Model file for the job. Use its own axes, mm. Round coordinates to 2 decimals unless told otherwise and drop trailing zeros. Loops run counter-clockwise (first coordinate to the right, second up) from the corner with the lowest first, then second, coordinate; pieces in that order, holes last. Notation, with made-up numbers: (59.25, 9.5) - (87.25, 9.5) arc R16 ccw to (87.25, 19.5) - close; hole circle Ø6 at (12.5, -1.75). An arc over 180 degrees is marked (long way). Answer as a JSON object with one key per item and string values.
from build123d import *

# Parameters (mm, degrees)
BOSS_EXTRUDE1_DEPTH = 3.175
CUT_EXTRUDE1_REACH  = 5.175
SKETCH2_R           = 7.14375
SKETCH3_R           = 6.35
CUT_EXTRUDE2_DEPTH  = 4.175


with BuildPart() as part:
    # Sketch1 → Boss-Extrude1 (new body)
    with BuildSketch(Plane(origin=(0, 0, 0), x_dir=(1, 0, 0), z_dir=(0, 1, 0))):
        Polygon((0, 0), (317.5, 0), (1073.15, 762), (-755.65, 762), align=None)
    extrude(amount=BOSS_EXTRUDE1_DEPTH)

    # Sketch2 → Cut-Extrude1 (cut, up to next)
    with BuildSketch(Plane(origin=(0, 3.175, 0), x_dir=(1, 0, 0), z_dir=(0, 1, 0)), mode=Mode.PRIVATE) as cut_extrude1_sk1:
        with Locations((-171.45, 419.1)):
            Circle(SKETCH2_R)
    cut_extrude1_tool1 = extrude(cut_extrude1_sk1.sketch, amount=-CUT_EXTRUDE1_REACH, mode=Mode.PRIVATE) & part.part
    add(cut_extrude1_tool1.solids().sort_by_distance((-171.45, 3.175, -419.1))[0], mode=Mode.SUBTRACT)
    # Sketch2 → Cut-Extrude1 (cut, up to next)
    with BuildSketch(Plane(origin=(0, 3.175, 0), x_dir=(1, 0, 0), z_dir=(0, 1, 0)), mode=Mode.PRIVATE) as cut_extrude1_sk2:
        with Locations((488.95, 419.1)):
            Circle(SKETCH2_R)
    cut_extrude1_tool2 = extrude(cut_extrude1_sk2.sketch, amount=-CUT_EXTRUDE1_REACH, mode=Mode.PRIVATE) & part.part
    add(cut_extrude1_tool2.solids().sort_by_distance((488.95, 3.175, -419.1))[0], mode=Mode.SUBTRACT)

    # Sketch3 → Cut-Extrude2 (cut, through all)
    with BuildSketch(Plane(origin=(0, 3.175, 0), x_dir=(1, 0, 0), z_dir=(0, 1, 0))):
        with Locations((-593.402017408, 634.460857891)):
            Circle(SKETCH3_R)
        with Locations((-450.320360604, 490.176834222)):
            Circle(SKETCH3_R)
        with Locations((-307.238703799, 345.892810554)):
            Circle(SKETCH3_R)
        with Locations((-164.157046994, 201.608786885)):
            Circle(SKETCH3_R)
        with Locations((481.657046994, 201.608786885)):
            Circle(SKETCH3_R)
        with Locations((624.738703799, 345.892810554)):
            Circle(SKETCH3_R)
        with Locations((767.820360604, 490.176834222)):
            Circle(SKETCH3_R)
        with Locations((910.902017408, 634.460857891)):
            Circle(SKETCH3_R)
    extrude(amount=-CUT_EXTRUDE2_DEPTH, mode=Mode.SUBTRACT)


solid = part.part
1) Slice it at C-C on x = -47. List the corners of the cut face in (y, z) (3 decimals), then the cut area to 3 significant figures.
Values follow:
{"outline": "(0, -762) - (3.175, -762) - (3.175, -47.395) - (0, -47.395) - close", "area": "2,270 mm²"}
2) Probe probe 1 along X at (y, z) = (1.25, -419.1); probe 2 along Z at (x, y) = (-171.45, 1.85); probe 3 along Z at (x, y) = (898, 2.15). List the from-to ranges inside material, lowest first.
Values follow:
{"probe 1": "-415.61 to -178.59, -164.31 to 481.81, 496.09 to 733.11", "probe 2": "-762 to -426.24, -411.96 to -172.89", "probe 3": "-762 to -585.38"}
3) Slice it at A-A on y = 0.9. Count the separate pieces of the cut face and the enclosed holes in it, then the cut area to 3 significant figures.
Values follow:
{"separate pieces": "1", "enclosed holes": "10", "area": "816,000 mm²"}
4) Slice it at B-B on x = 371. List the corners of the cut face in (y, z) (3 decimals), then the cut area to 3 significant figures.
Values follow:
{"outline": "(0, -762) - (3.175, -762) - (3.175, -53.95) - (0, -53.95) - close", "area": "2,250 mm²"}
5) Drop flat-ended pins along their axis: P1, Ø1.5, axis at x = -346, y = 0.5, coming from the +Z side; P2, Ø1.5, axis at y = 1.5, z = -194.5, coming from the -X side. Give the stop position or say it passes through.
Values follow:
{"P1": "z = -348.15", "P2": "x = -193.62"}
